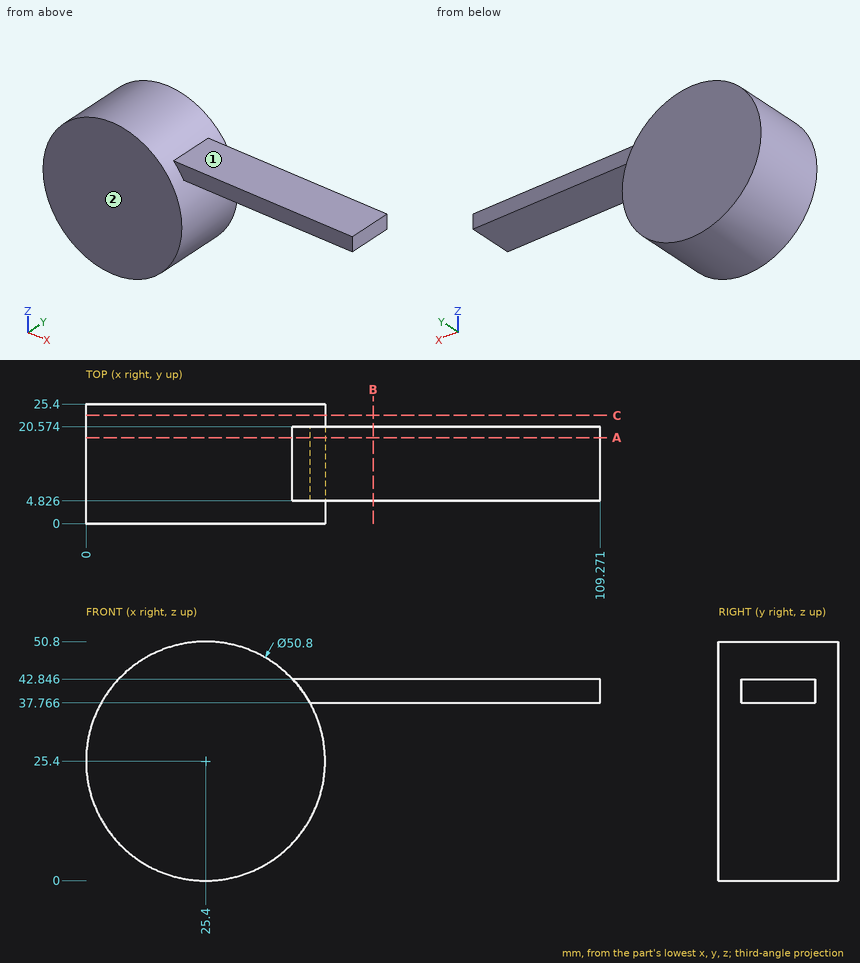
Can you work these out from the drawing? Everything is in mm from the part's minimum corner. A direction names the side the tool comes from. Round coordinates to 2 decimals unless told otherwise and drop trailing zeros. Write each loop counter-clockwise with the first axis right and the second up, starting at its lowest first coordinate (ties: lowest second). Pieces come first, ordered by that corner, then holes. Notation, with made-up numbers: (-14, 21) - (-10, 21) arc R29 cw to (-10, 41) - close; hole circle Ø10 at (-2, 88). An arc over 180 degrees is marked (long way). Put each result on its own line as item: value. Start each with the question number.
(1) I need wall thicknesses on probe 1 along Z at (x, y) = (59, 17.75); probe 2 along Y at (x, z) = (56.5, 42); probe 3 along X at (y, z) = (24.75, 26). Which ranges of each line are inside material? Lowest first, please.
(2) I want a section at A-A, the plane y = 18.25. Please give me the cut outline in (x, z).
(3) Will these pins go through, and if not, where does the flat tip stop? pin 1 (8 mm diameter, centred on y = 16.5, z = 14.5, fed in from -X) (1 decimal); pin 2 (3 mm diameter, centred on x = 92.5, y = 4.5, fed in from +Z); pin 3 (1 mm diameter, centred on y = 3.5, z = 44, fed in from +X); pin 4 (6 mm diameter, centred on y = 10, z = 45, fed in from +X).
(4) For the marked faces 1 and 2, which set-ups out of +Z, -Z, +X, -X, +Y, -Y let a thin tool reach every point of the face, with its end or its side?
(5) I want a section at C-C, the plane y = 23. Please give me the cut outline in (x, z).
(6) I want a section at B-B, the plane x = 61. Please give me the cut outline in (y, z), plus the area to 3 significant figures.
Here are the results:
1. probe 1: z = 37.77 to 42.85
1. probe 2: y = 4.83 to 20.57
1. probe 3: x = 0.01 to 50.79
2. outline: (43.86, 42.85) arc R25.4 ccw (long way) to (47.59, 37.77) - (109.27, 37.77) - (109.27, 42.85) - close
3. pin 1: stops at x = 1
3. pin 2: stops at z = 42.85
3. pin 3: stops at x = 43.22
3. pin 4: stops at x = 109.27
4. face 1: +Z, +X, +Y, -Y
4. face 2: +Z, -Z, +X, -X, -Y
5. outline: circle Ø50.8 at (25.4, 25.4)
6. outline: (4.83, 37.77) - (20.57, 37.77) - (20.57, 42.85) - (4.83, 42.85) - close
6. area: 80.0 mm^2
